```python
from build123d import *

# Parameters (mm, degrees)
ESQUISSE1_W        = 250
ESQUISSE1_H        = 100
ESQUISSE1_R        = 10
BOSS_EXTRU_1_DEPTH = 140


with BuildPart() as part:
    # Esquisse1 → Boss.-Extru.1 (new body)
    with BuildSketch(Plane.XY):
        Rectangle(ESQUISSE1_W, ESQUISSE1_H)
        with Locations((-83.402754161, 33.361101664)):
            Circle(ESQUISSE1_R, mode=Mode.SUBTRACT)
        with Locations(Location((83.402754161, 33.361101664, 0), (0, 0, 180))):
            Circle(ESQUISSE1_R, mode=Mode.SUBTRACT)
        with Locations((83.402754161, -33.361101664)):
            Circle(ESQUISSE1_R, mode=Mode.SUBTRACT)
        with Locations(Location((-83.402754161, -33.361101664, 0), (0, 0, 180))):
            Circle(ESQUISSE1_R, mode=Mode.SUBTRACT)
        with BuildLine():
            Line((-33.78724139, 17.132226308), (35.196852355, 17.132226308))
            ThreePointArc((35.196852355, 17.132226308), (52.329078664, 0), (35.196852355, -17.132226308))
            Line((35.196852355, -17.132226308), (-33.78724139, -17.132226308))
            ThreePointArc((-33.78724139, -17.132226308), (-50.919467698, 0), (-33.78724139, 17.132226308))
        make_face(mode=Mode.SUBTRACT)
    extrude(amount=BOSS_EXTRU_1_DEPTH)


solid = part.part
```
Geometry check sheet. Reference: the model listing, model coordinates, mm. A direction names the side the tool comes from. Round coordinates to 2 decimals unless told otherwise and drop trailing zeros. Order: outer loops, then holes, each group sorted by start corner. A loop starts at its lowest first (then second) coordinate and runs counter-clockwise, first axis right, second up. Notation, with made-up numbers: (-32, -17) - (5, -17) arc R26 ccw to (5, 6) - close; hole circle Ø9 at (-5.75, 42). An arc over 180 degrees is marked (long way). Use a Markdown table: item, result. Add a question column.
(1) Depth check by flat-ended pin: pin 1 (10 mm diameter, centred on x = -5, y = -14.5, fed in from +Z). Enter the tip coordinate at first touch or a pass-through.
(2) Sectioned sample at B-B, the plane y = 0. Enter the section's corners in (x, z).
(3) Tool access check on faces 1 (the flat face through (0, 17.132, 69)), 2 (the flat face through (-2, 23, 0)). Record the directions out of +Z, -Z, +X, -X, +Y, -Y that give a thin tool (end or side, any length) a straight path to the whole face; none if there is none.
(4) Sectioned sample at C-C, the plane z = 92.5. Enter the section's corners in (x, y), and give its area (3 significant figures).
(5) Sectioned sample at D-D, the plane y = -28.5. Enter the section's corners in (x, z), and give its area (3 significant figures).
(6) Release check for a two-part mould opening along Y. For faces 3 (the flat face through (-125, -1, 69)), 4 (the cylindrical face through (92.94, -30.36, 69.02)), 5 (the flat face through (-2, -50, 69)) record: pulls with the +Y half, pulls with the -Y half, needs draft (parallel to the pull), parting line crosses it, or undercut.
(7) Material ranges on line 1 along Y through (x, z) = (-83.5, 74.5); line 2 along X through (y, z) = (-32.5, 73); line 3 along X through (y, z) = (-41, 90), recorded low to high. Write a range as [from, to].
(8) Sectioned sample at A-A, the plane x = 0. Enter the section's corners in (y, z), and give its area (3 significant figures).
Answers below:
| question | item | result |
|---|---|---|
| 1 | pin 1 | z = 140 |
| 2 | outline | (-125, 0) - (-50.92, 0) - (-50.92, 140) - (-125, 140) - close; (52.33, 0) - (125, 0) - (125, 140) - (52.33, 140) - close |
| 3 | face 1 | +Z, -Z |
| 3 | face 2 | -Z, +X, -X, +Y, -Y |
| 4 | outline | (-125, -50) - (125, -50) - (125, 50) - (-125, 50) - close; hole circle Ø20 at (-83.4, -33.36); hole circle Ø20 at (-83.4, 33.36); hole (-33.79, -17.13) - (35.2, -17.13) arc R17.13 ccw to (35.2, 17.13) - (-33.79, 17.13) arc R17.13 ccw to start; hole circle Ø20 at (83.4, -33.36); hole circle Ø20 at (83.4, 33.36) |
| 4 | area | 20,500 mm² |
| 5 | outline | (-125, 0) - (-92.14, 0) - (-92.14, 140) - (-125, 140) - close; (-74.66, 0) - (74.66, 0) - (74.66, 140) - (-74.66, 140) - close; (92.14, 0) - (125, 0) - (125, 140) - (92.14, 140) - close |
| 5 | area | 30,100 mm² |
| 6 | face 3 | needs draft |
| 6 | face 4 | undercut |
| 6 | face 5 | pulls with the -Y half |
| 7 | line 1 | [-50, -43.36], [-23.36, 23.36], [43.36, 50] |
| 7 | line 2 | [-125, -93.37], [-73.44, 73.44], [93.37, 125] |
| 7 | line 3 | [-125, -89.86], [-76.95, 76.95], [89.86, 125] |
| 8 | outline | (-50, 0) - (-17.13, 0) - (-17.13, 140) - (-50, 140) - close; (17.13, 0) - (50, 0) - (50, 140) - (17.13, 140) - close |
| 8 | area | 9,200 mm² |
